Input: part model. Units: mm. Frame: model coordinates. A direction names the side the tool comes from. Round coordinates to 2 decimals unless told otherwise and drop trailing zeros.
(1) First-contact query: pin 1 Ø1.5 at (y, z) = (-4.5, -15) entering from -X; pin 2 Ø5.5 at (x, z) = (9.24, -16) entering from -Y; pin 3 Ø9.5 at (x, z) = (-2.26, -5) entering from -Y. Flat tips, straight axial feed; report the tip coordinate or a pass-through.
(2) Access query for faces 1 (the face through (11, -2, -17)), 2 (the face through (10, 0, 0)). Directions: +Z, -Z, +X, -X, +Y, -Y. A direction counts if a zero-diameter tool reaches every point of the face in a straight line with its end or side. Return the directions, or none.
(3) Line query: line 1 (Y direction, x = -3.5, z = -11); line 2 (Z direction, x = 8, y = -1.5); line 3 (Z direction, x = 10, y = -2.75). Output: solid intervals per line, ascending.
(4) Draft query along Z for faces 3 (the face through (34.026, -4.196, -0.07)), 4 (the face through (0.8, -3.46, -12.39)), 5 (the face through (9.076, -2.476, -19.465)), 6 (the face through (8.336, -3.528, 13.139)). Return one class per face: released by +Z, released by -Z, zero draft, split by the parting line, or undercut.
Solid Edge part; units mm, degrees
sketch "Sketch1" plane through (0, 0, 0) normal (0, -1, 0) x (1, 0, 0)
  line L0 (35.7368, 5) -> (35.7368, -5)
  line L1 (20.7368, -20) -> (-2.2632, -20)
  line L2 (-17.2632, 5) -> (-17.2632, -5)
  line L3 (20.7368, 20) -> (-2.2632, 20)
  arc A0 (35.7368, -5) -> (20.7368, -20) centre (20.7368, -5) cw
  arc A1 (-2.2632, -20) -> (-17.2632, -5) centre (-2.2632, -5) cw
  arc A2 (-17.2632, 5) -> (-2.2632, 20) centre (-2.2632, 5) cw
  arc A3 (20.7368, 20) -> (35.7368, 5) centre (20.7368, 5) cw
extrude "Protrusion1" add sketch "Sketch1" along normal blind 6
fillet "Redondeo_1" radius 6 8 edges at (31.3434, -6, 15.6066) (35.7368, -6, 0) (31.3434, -6, -15.6066) (9.2368, -6, -20) (-12.8698, -6, -15.6066) (-17.2632, -6, 0) (-12.8698, -6, 15.6066) (9.2368, -6, 20)
hole "Agujero_1" at (-2.2632, -6, -5) direction (0, 1, 0) diameter 9 end up to next counterbore diameter 16 counterbore depth 5
hole "Agujero_2" at (9.2368, -6, 16) direction (0, 1, 0) diameter 3.5 end up to next counterbore diameter 6 counterbore depth 4
hole "Hole1" at (9.2368, -6, -16) direction (0, 1, 0) diameter 3.5 end up to next counterbore diameter 6 counterbore depth 4
hole "Hole2" at (29.3368, -6, 9.67) direction (0, 1, 0) diameter 3.5 end up to next counterbore diameter 6 counterbore depth 4
Reported:
1. pin 1: stops at x = -11.89
1. pin 2: stops at y = -2
1. pin 3: stops at y = -1
2. face 1: -Y
2. face 2: +Z, -Z, +X, -X, +Y
3. line 1: y = -1 to 0
3. line 2: z = -19.81 to -17.24, -14.76 to 14.76, 17.24 to 19.81
3. line 3: z = -19.33 to -18.9, -13.1 to 13.1, 18.9 to 19.33
4. face 3: zero draft
4. face 4: undercut
4. face 5: released by -Z
4. face 6: undercut
